Verification items for the finished model (mm, model axes). A direction names the side the tool comes from. Coordinates: 2 decimals unless noted, no trailing zeros. Order: outer loops, then holes, each group sorted by start corner. A loop starts at its lowest first (then second) coordinate and runs counter-clockwise, first axis right, second up.
Q1. Cross-section at A-A, the plane x = -5.5. Record the boundary of the cut face in (y, z).
Q2. Thickness scan on line 1 (X direction, y = 10, z = 36); line 2 (Y direction, x = -5.5, z = 57); line 3 (Z direction, x = 7, y = 7). Record the ranges inside material, lowest first.
Q3. Cross-section at B-B, the plane z = 51.5. Record the boundary of the cut face in (x, y).
Q4. Cross-section at D-D, the plane y = 7.5. Count the separate pieces of the cut face and the enclosed holes in it, and give its area (3 significant figures).
Q5. Set-up check for faces 3 (the cylindrical face through (12.857, 6.753, 36.451)), 4 (the flat face through (4, 0.5, 64)), 5 (the flat face through (-3.8, 9.2, 55)), 6 (the flat face through (4.5, 8, 64)), 7 (the flat face through (9, 10, 4)): record each of +Z, -Z, +X, -X, +Y, -Y from which the full face is reachable in a straight line by a thin tool's end or side.
Q6. Cross-section at C-C, the plane x = 21.5. Record the boundary of the cut face in (y, z), and give its area (4 significant figures).
Q7. Draft check along X on faces 1 (the flat face through (9, 7, 8)), 2 (the conical face through (4.44, 9.927, 41.614)). Enter one of: pulls with the +X half, pulls with the -X half, needs draft (parallel to the pull), parting line crosses it, or undercut.
Q8. Depth check by flat-ended pin: P1, Ø5, axis at y = 9.5, z = 34, coming from the -X side; P2, Ø5, axis at y = 3, z = 46.5, coming from the +X side; P3, Ø1.2, axis at x = 9, z = 3.5, coming from the +Y side. Enter the tip coordinate at first touch or a pass-through.
from build123d import *

# Parameters (mm, degrees)
SKETCH_1_W             = 18
SKETCH_1_H             = 10
EXTRUDE_1_DEPTH        = 65
SKETCH_2_W             = 25
SKETCH_2_H             = 5
CUT_EXTRUDE_1_DEPTH    = 69.183575735
SKETCH_3_W             = 18
SKETCH_3_H             = 32
EXTRUDE_2_DEPTH        = 5
SKETCH_4_W             = 38
SKETCH_4_H             = 10
EXTRUDE_3_DEPTH        = 15
HOLE_WIZARD_M5_1_D     = 4.2
PATTERN_LINEAR_2_COUNT = 2
PATTERN_LINEAR_2_PITCH = 8
CUT_EXTRUDE_2_DEPTH    = 73.346388991
CHAMFER_1_SIZE         = 0.5
SKETCH_10_W            = 12
SKETCH_10_H            = 77.617391284
CUT_EXTRUDE_3_DEPTH    = 0.5


with BuildPart() as part:
    # 草图1 → 凸台-拉伸1 (new body)
    with BuildSketch(Plane.XY):
        with Locations((9, 5)):
            Rectangle(SKETCH_1_W, SKETCH_1_H)
    extrude(amount=EXTRUDE_1_DEPTH)

    # 草图2 → 切除-拉伸1 (cut, through all)
    with BuildSketch(Plane.ZY):
        with Locations((20.5, 7.5)):
            Rectangle(SKETCH_2_W, SKETCH_2_H)
    extrude(amount=-CUT_EXTRUDE_1_DEPTH, mode=Mode.SUBTRACT)

    # 草图3 → 凸台-拉伸2 (add)
    with BuildSketch(Plane(origin=(0, 10, 0), x_dir=(1, 0, 0), z_dir=(0, 1, 0))):
        with Locations((9, -49)):
            Rectangle(SKETCH_3_W, SKETCH_3_H)
    extrude(amount=EXTRUDE_2_DEPTH)

    # 草图4 → 凸台-拉伸3 (add)
    with BuildSketch(Plane(origin=(0, 15, 0), x_dir=(1, 0, 0), z_dir=(0, 1, 0))):
        with Locations((9, -60)):
            Rectangle(SKETCH_4_W, SKETCH_4_H)
    extrude(amount=-EXTRUDE_3_DEPTH)

    # M5 螺纹孔1 (through all)
    with Locations(Plane.XY.offset(65)):
        with Locations((-5.5, 7.5)):
            Hole(HOLE_WIZARD_M5_1_D / 2)

    # 草图7 → Ø6.5 (6.5) 直径孔1 (revolve, cut)
    with BuildSketch(Plane(origin=(13, 10, 0), x_dir=(0, 1, 0), z_dir=(1, 0, 0))):
        Polygon((0, 0), (0, 41.952797012), (3.25, 40), (3.25, 0), align=None)
    hole_wizard_6_5_6_5_1 = revolve(axis=Axis((13, 10, -6.35), (0, 0, 1)), mode=Mode.SUBTRACT)

    # 阵列(线性)2: Ø6.5 (6.5) 直径孔1 ×2
    with Locations(*[(-i * PATTERN_LINEAR_2_PITCH, 0, 0) for i in range(1, PATTERN_LINEAR_2_COUNT)]):
        add(hole_wizard_6_5_6_5_1, mode=Mode.SUBTRACT)

    # 草图9 → 切除-拉伸2 (cut, through all)
    with BuildSketch(Plane(origin=(0, 15, 0), x_dir=(1, 0, 0), z_dir=(0, 1, 0))):
        with BuildLine():
            Line((13.5, -65), (4.5, -65))
            Line((4.5, -65), (4.5, -62.2))
            Line((4.5, -62.2), (2, -62.2))
            ThreePointArc((2, -62.2), (1.646446609, -62.053553391), (1.5, -61.7))
            Line((1.5, -61.7), (1.5, -59.2))
            ThreePointArc((1.5, -59.2), (1.646446609, -58.846446609), (2, -58.7))
            Line((2, -58.7), (16, -58.7))
            ThreePointArc((16, -58.7), (16.353553391, -58.846446609), (16.5, -59.2))
            Line((16.5, -59.2), (16.5, -61.7))
            ThreePointArc((16.5, -61.7), (16.353553391, -62.053553391), (16, -62.2))
            Line((16, -62.2), (13.5, -62.2))
            Line((13.5, -62.2), (13.5, -65))
        make_face()
    extrude(amount=-CUT_EXTRUDE_2_DEPTH, mode=Mode.SUBTRACT)

    # 倒角1
    chamfer_1_edges = [part.edges().sort_by_distance(p)[0] for p in [
        (20.75, 15, 65),
        (20.75, 0, 65),
        (13.5, 0, 63.6),
        (4.5, 0, 63.6),
        (3.25, 0, 62.2),
        (1.646446609, 0, 62.053553391),
        (1.5, 0, 60.45),
        (1.646446609, 0, 58.846446609),
        (9, 0, 58.7),
        (16.353553391, 0, 58.846446609),
        (16.5, 0, 60.45),
        (16.353553391, 0, 62.053553391),
        (14.75, 0, 62.2),
        (13.5, 15, 63.6),
        (14.75, 15, 62.2),
        (16.353553391, 15, 62.053553391),
        (16.5, 15, 60.45),
        (16.353553391, 15, 58.846446609),
        (9, 15, 58.7),
        (1.646446609, 15, 58.846446609),
        (1.5, 15, 60.45),
        (1.646446609, 15, 62.053553391),
        (3.25, 15, 62.2),
        (4.5, 15, 63.6),
        (9, 15, 33),
        (0, 15, 44),
        (-2.75, 15, 65),
        (18, 15, 44),
        (18, 0, 27.5),
        (0, 0, 27.5),
        (-5, 15, 55),
        (-10, 15, 60),
        (23, 15, 55),
        (28, 15, 60),
        (-5, 0, 55),
        (-10, 0, 60),
        (23, 0, 55),
        (28, 0, 60),
        (-10, 7.5, 55),
        (28, 7.5, 65),
        (-10, 7.5, 65),
        (28, 7.5, 55),
        (9, 0, 0),
        (-2.75, 0, 65),
    ]]
    chamfer(chamfer_1_edges, length=CHAMFER_1_SIZE)

    # 草图10 → 切除-拉伸3 (cut)
    with BuildSketch(Plane.XZ):
        with Locations((9, 33.316007813)):
            Rectangle(SKETCH_10_W, SKETCH_10_H)
    extrude(amount=-CUT_EXTRUDE_3_DEPTH, mode=Mode.SUBTRACT)


solid = part.part
Check values:
1. outline: (0, 55.5) - (0.5, 55) - (5.4, 55) - (5.4, 65) - (0.5, 65) - (0, 64.5) - close; (9.6, 55) - (14.5, 55) - (15, 55.5) - (15, 64.5) - (14.5, 65) - (9.6, 65) - close
2. line 1: x = 0 to 1.75, 8.25 to 9.75, 16.25 to 18
2. line 2: y = 0 to 5.4, 9.6 to 15
2. line 3: z = 0 to 8, 33 to 58.7
3. outline: (0, 0.5) - (0.5, 0) - (3, 0) - (3, 0.5) - (15, 0.5) - (15, 0) - (17.5, 0) - (18, 0.5) - (18, 14.5) - (17.5, 15) - (0.5, 15) - (0, 14.5) - close
4. separate pieces: 5
4. enclosed holes: 0
4. area: 673 mm2
5. face 3: -Z
5. face 4: +Z, -Z, -Y
5. face 5: -Z, -X, +Y, -Y
5. face 6: +Z, +Y, -Y
5. face 7: -Z, +X, -X, +Y
6. outline: (0, 55.5) - (0.5, 55) - (14.5, 55) - (15, 55.5) - (15, 64.5) - (14.5, 65) - (0.5, 65) - (0, 64.5) - close
6. area: 149.5 mm2
7. face 1: needs draft
7. face 2: undercut
8. P1: stops at x = 0
8. P2: stops at x = 18
8. P3: stops at y = 10
